```python
from build123d import *

# Parameters (mm, degrees)
SKETCH_2_R               = 5
CUT_EXTRUDE_1_DEPTH      = 49.84301383
CUT_EXTRUDE_START        = -8
SKETCH_3_R               = 8
CUT_EXTRUDE_2_DEPTH      = 8
CHAMFER_1_SIZE2          = 1.732050808
CHAMFER_1_SIZE           = 3
HOLE_WIZARD_M5_1_D       = 4.2
CUT_EXTRUDE_3_DEPTH      = 48.428261617
PATTERN_CIRCULAR_1_COUNT = 3
CHAMFER_4_SIZE           = 0.5
EXTRUDE_START            = 12
EXTRUDE_1_DEPTH          = 12
CHAMFER_5_SIZE           = 1.5
CHAMFER_6_SIZE           = 0.5
FILLET_1_R               = 0.2


# Some blends are built 0.0001 mm under size
with BuildPart() as part:
    # 草图1 → 旋转1 (revolve)
    with BuildSketch(Plane.XY, mode=Mode.PRIVATE) as revolve_1_sk:
        Polygon((0, 0), (0, 10), (3, 10), (3, 30), (8, 30), (8, 9.6), (11, 9.6), (11, 8.5), (21.2, 8.5), (21.2, 8), (22.2, 8), (22.2, 8.4), (24.2, 8.4), (24.2, 0), align=None)
    revolve(revolve_1_sk.sketch.rotate(Axis((24.2, 0, 0), (-1, 0, 0)), 90), axis=Axis((24.2, 0, 0), (-1, 0, 0)))

    # 草图2 → 切除-拉伸1 (cut, through all)
    with BuildSketch(Plane(origin=(24.2, 0, 0), x_dir=(0, 0, -1), z_dir=(1, 0, 0))):
        Circle(SKETCH_2_R)
    extrude(amount=-CUT_EXTRUDE_1_DEPTH, mode=Mode.SUBTRACT)

    # 草图3 → 切除-拉伸2 (cut)
    with BuildSketch(Plane.ZY.offset(CUT_EXTRUDE_START)):
        with Locations(Location((0, 0, 0), (0, 0, 180))):
            Circle(SKETCH_3_R)
    extrude(amount=CUT_EXTRUDE_2_DEPTH, mode=Mode.SUBTRACT)

    # 倒角1
    chamfer_1_edges = [part.edges().sort_by_distance(p)[0] for p in [
        (8, 0, 5),
    ]]
    chamfer_1_side = [part.faces().sort_by_distance(p)[0] for p in [
        (8, 0, 5.034641016),
    ]]
    chamfer(chamfer_1_edges, length=CHAMFER_1_SIZE - 0.0001, length2=CHAMFER_1_SIZE2 - 0.0001, reference=chamfer_1_side[0])  # a hair under: the kernel refuses the full size

    # M5 螺纹孔1 (through all)
    with Locations(Plane(origin=(3, 25, 0), x_dir=(0, 0, -1), z_dir=(-1, 0, 0))):
        with Locations((0, 0), (-21.650635095, 37.5), (21.650635095, 37.5)):
            Hole(HOLE_WIZARD_M5_1_D / 2)

    # 草图4 → 切除-拉伸3 (cut, through all)
    with BuildSketch(Plane.ZY.offset(-3)):
        with BuildLine():
            ThreePointArc((-27.710194429, -21.380952381), (0, -35), (27.710194429, -21.380952381))
            ThreePointArc((27.710194429, -21.380952381), (0, -13), (-27.710194429, -21.380952381))
        make_face()
    cut_extrude_3 = extrude(amount=-CUT_EXTRUDE_3_DEPTH, mode=Mode.SUBTRACT)

    # 阵列(圆周)1: 切除-拉伸3 ×3 about axis
    pattern_circular_1_axis = Axis((0, 0, 0), (1, 0, 0))
    for i in range(1, PATTERN_CIRCULAR_1_COUNT):
        add(cut_extrude_3.rotate(pattern_circular_1_axis, i * 360 / PATTERN_CIRCULAR_1_COUNT), mode=Mode.SUBTRACT)

    # 倒角2
    # the kernel refuses this chamfer: 1.262336382, 1 mm, written as the material it takes off along each edge
    with BuildSketch(Plane(origin=(-0.323534522, -18.801587302, -23.377346191), x_dir=(0, 0.7894182220381707, -0.6138557409637001), z_dir=(1, 0, 0)), Plane(origin=(-0.323534522, -10.844582024, 27.97132533), x_dir=(0, -0.9263237769525716, -0.3767283640135453), z_dir=(1, 0, 0)), Plane(origin=(-0.323534522, 29.646169325, -4.593979139), x_dir=(0, 0.13690555491440626, 0.9905841049772496), z_dir=(1, 0, 0))) as chamfer_2_piece_1:
        with BuildLine():
            Line((0.983994902, 0), (-0.239625676, 1.264429883))
            ThreePointArc((-0.239625676, 1.264429883), (-0.119678092, 0.653717986), (0, 0))
            ThreePointArc((0, 0), (0.509546154, -0.004029497), (0.983994902, 0))
        make_face()
    extrude(amount=11.647069044, mode=Mode.SUBTRACT)
    with BuildSketch(Plane(origin=(-0.323534522, -10.844582024, -27.97132533), x_dir=(0, 0.5426204152715339, 0.8399780264569711), z_dir=(1, 0, 0)), Plane(origin=(-0.323534522, 29.646169325, 4.593979139), x_dir=(0, -0.9987525171682211, 0.04993405100872917), z_dir=(1, 0, 0))) as chamfer_2_piece_2:
        with BuildLine():
            Line((1.28693566, 0), (-0.183218517, 0.966786917))
            ThreePointArc((-0.183218517, 0.966786917), (-0.098835833, 0.499884984), (0, 0))
            ThreePointArc((0, 0), (0.664569743, 0.004136227), (1.28693566, 0))
        make_face()
    extrude(amount=11.647069044, mode=Mode.SUBTRACT)
    with BuildSketch(Plane(origin=(-0.323534522, -18.801587302, 23.377346191), x_dir=(0, 0.7894182220381672, 0.6138557409637047), z_dir=(1, 0, 0))) as chamfer_2_piece_3:
        with BuildLine():
            Line((0.983994902, 0), (-0.239625676, -1.264429883))
            ThreePointArc((-0.239625676, -1.264429883), (-0.119678092, -0.653717986), (0, 0))
            ThreePointArc((0, 0), (0.509546154, 0.004029497), (0.983994902, 0))
        make_face()
    extrude(amount=11.647069044, mode=Mode.SUBTRACT)

    # 倒角4
    chamfer_4_edges = [part.edges().sort_by_distance(p)[0] for p in [
        (0, 0, 10),
    ]]
    chamfer(chamfer_4_edges, length=CHAMFER_4_SIZE)

    # 草图7 → 凸台-拉伸1 (add)
    with BuildSketch(Plane(origin=(24.2, 0, 0), x_dir=(0, 0, -1), z_dir=(1, 0, 0)).offset(EXTRUDE_START)):
        with BuildLine():
            Line((-6.8, -6), (6.8, -6))
            Line((6.8, -6), (6.8, 4.769696007))
            Line((6.8, 4.769696007), (1.5, 4.769696007))
            ThreePointArc((1.5, 4.769696007), (0, -5), (-1.5, 4.769696007))
            Line((-1.5, 4.769696007), (-6.8, 4.769696007))
            Line((-6.8, 4.769696007), (-6.8, -6))
        make_face()
    extrude(amount=-EXTRUDE_1_DEPTH)

    # 倒角5
    # the kernel refuses this chamfer: 1.5 mm, written as the material it takes off along each edge
    with BuildSketch(Plane(origin=(40.057524482, 4.769696007, 6.8), x_dir=(0, 0, -1), z_dir=(-1, 0, 0)), Plane(origin=(40.057524482, -6, 6.8), x_dir=(0, 1, 0), z_dir=(-1, 0, 0))) as chamfer_5_piece_1:
        Polygon((CHAMFER_5_SIZE, 0), (0, CHAMFER_5_SIZE), (0, 0), align=None)
    extrude(amount=15.857524482, mode=Mode.SUBTRACT)
    with BuildSketch(Plane(origin=(40.057524482, -6, -6.8), x_dir=(0, 1, 0), z_dir=(-1, 0, 0)), Plane(origin=(40.057524482, 4.769696007, -6.8), x_dir=(0, 0, 1), z_dir=(-1, 0, 0))) as chamfer_5_piece_2:
        Polygon((CHAMFER_5_SIZE, 0), (0, -CHAMFER_5_SIZE), (0, 0), align=None)
    extrude(amount=15.857524482, mode=Mode.SUBTRACT)

    # 倒角6
    chamfer_6_edges = [part.edges().sort_by_distance(p)[0] for p in [
        (36.2, -5, 0),
    ]]
    chamfer(chamfer_6_edges, length=CHAMFER_6_SIZE)

    # 圆角1
    # the kernel refuses this fillet: 0.2 mm, written as the material it takes off along each edge
    with BuildSketch(Plane(origin=(38.153768211, 4.769696007, 1.5), x_dir=(0, -0.3904189103265273, 0.9206373197190341), z_dir=(-1, 0, 0))) as fillet_1_piece_1:
        with BuildLine():
            CenterArc((0.981696018, 0.199071541), FILLET_1_R, 112.980567733, 151.496467657)
            Line((0.903612236, 0.383199004), (0, 0))
            ThreePointArc((0, 0), (0.481223538, 0.023211487), (0.962447076, 0))
        make_face()
    extrude(amount=13.953768211, mode=Mode.SUBTRACT)
    with BuildSketch(Plane(origin=(38.153768211, 4.769696007, -1.5), x_dir=(0, -0.39041891032652715, -0.9206373197190343), z_dir=(-1, 0, 0))) as fillet_1_piece_2:
        with BuildLine():
            CenterArc((0.981696018, -0.199071541), FILLET_1_R, 95.52296461, 151.496467657)
            Line((0.903612236, -0.383199004), (0, 0))
            ThreePointArc((0, 0), (0.481223538, -0.023211487), (0.962447076, 0))
        make_face()
    extrude(amount=13.953768211, mode=Mode.SUBTRACT)


solid = part.part
```
Design review of the part built by this model. Coordinates are the model's own, in mm. A direction names the side the tool comes from. Coordinates: 2 decimals unless noted, no trailing zeros. Order: outer loops, then holes, each group sorted by start corner. A loop starts at its lowest first (then second) coordinate and runs counter-clockwise, first axis right, second up. Notation, with made-up numbers: M 42,11 L 64,11 A19 cw 64,47 Z; hole C -30.75,7 d7. An arc over 180 degrees is marked long. Answer as a JSON object with one key per item and string values. Group by question number.
1) Add section C-C, the plane x = 13. Write out the cut boundary in (y, z), then the cut area to 3 significant figures.
2) Tool access review of faces 1 (the cylindrical face through (2, 0, 10)), 2 (the flat face through (30, -6, 0)), 3 (the cylindrical face through (16.171, -8.428, 1.107)), 4 (the flat face through (30, 4.77, 4)), 5 (the flat face through (30.3, -5.2, 6.1)): name each direction out of +Z, -Z, +X, -X, +Y, -Y from which nothing blocks a thin tool from reaching the whole face with its end or side.
3) For pin 1 (6 mm diameter, centred on x = 23.5, z = -7.5, fed in from +Y); pin 2 (8 mm diameter, centred on x = 19.5, z = 7, fed in from +Y); pin 3 (6 mm diameter, centred on x = 32.5, y = -1, fed in from -Z), all flat-tipped, find the tip position at first contact; note any pin that passes through.
4) Add section D-D, the plane z = -1. Count the separate pieces of the cut face and the enclosed holes in it, then the cut area to 3 significant figures.
5) Add section B-B, the plane z = -20.5. Write out the cut boundary in (x, y), then the cut area to 3 significant figures.
6) Wall thickness on L1, parallel to Z at x = 29, y = 0; L2, parallel to Y at x = 18, z = 0; L3, parallel to X at y = -1, z = 8: over which ranges is each line inside the solid? List them lowest first.
7) Add section A-A, the plane y = 25. Write out the cut boundary in (x, z), then the cut area to 3 significant figures.
8) Mouldability with a two-part tool opening along Y and no side actions: class faces 6 (the conical face through (9.65, -5.02, 1.12)), 7 (the flat face through (30.28, 4.03, 6.04)), 8 (the cylindrical face through (4.06, 7.81, 1.73)), 9 (the cylindrical face through (5.535, -15.044, 25.955)) as pulls with the +Y half, pulls with the -Y half, needs draft (parallel to the pull), parting line crosses it, or undercut.
Computed values:
{
 "1": {"outline": "C 0,0 d17; hole C 0,0 d10", "area": "148 mm^2"},
 "2": {"face 1": "-X", "face 2": "+Z, -Z, +X, -Y", "face 3": "+X", "face 4": "+Z, -Z, +X, +Y", "face 5": "+Z, +X, -Y"},
 "3": {"pin 1": "stops at y = 7.09", "pin 2": "stops at y = 7.95", "pin 3": "stops at z = -6.8"},
 "4": {"separate pieces": "3", "enclosed holes": "0", "area": "257 mm^2"},
 "5": {"outline": "M 3,-17.4 L 8,-17.4 L 8,-14.26 L 3,-14.26 Z; M 3,-10.74 L 8,-10.74 L 8,-5.11 L 3,-5.11 Z", "area": "43.9 mm^2"},
 "6": {"L1": "z = -6.8 to -5, 5 to 6.8", "L2": "y = -8.5 to -5, 5 to 8.5", "L3": "x = 0 to 21.2, 22.2 to 24.2"},
 "7": {"outline": "M 3,-4.98 L 8,-4.98 L 8,-2.1 L 3,-2.1 Z; M 3,2.1 L 8,2.1 L 8,4.98 L 3,4.98 Z", "area": "28.8 mm^2"},
 "8": {"face 6": "undercut", "face 7": "pulls with the +Y half", "face 8": "undercut", "face 9": "pulls with the -Y half"}
}
